from build123d import *

# Parameters (mm, degrees)
F0_R         = 1.75
F1_DEPTH     = 4
F2_W         = 50
F2_H         = 3
F3_DEPTH     = 35
F4_R         = 1.75
F5_DEPTH     = 3
F6_T1_DEPTH  = 4
F6_T6_DEPTH  = 28.6040226041
F6_T13_DEPTH = 28.6040226041
F6_S15_R     = 1.75
F6_T16_DEPTH = 16
F6_T19_DEPTH = 15.1872089077
F6_T26_DEPTH = 13.4620824192
F6_T30_DEPTH = 28.6040226041
F6_S32_R     = 1.75
F6_T33_DEPTH = 16
F7_R         = 3.25
F7_R_2       = 1.75
F8_DEPTH     = 2
F9_SIZE      = 2


# Not quite as in the source:
# - a fillet or chamfer that OpenCascade refuses, or shapes differently, is made with other operations: its cross-section is extruded or revolved along the edge and cut away or added


with BuildPart() as f1:
    # F0 (on Top) → F1 (new body)
    with BuildSketch(Plane.XY):
        Polygon((-4.0152793502, 1.5), (-25, 1.5), (-25, -1.5), (25, -1.5), (25, 1.5), (4.0152793502, 1.5), align=None)
        Polygon((-1.8013300137, 26.8055567119), (-4.0152793502, 1.5), (4.0152793502, 1.5), (6.1682275711, 26.10831077), align=None)
        with BuildLine():
            Line((-12.7594716927, 27.7642698822), (-1.8013300137, 26.8055567119))
            Line((-1.8013300137, 26.8055567119), (-1.4744959784, 30.5412868298))
            Line((-1.4744959784, 30.5412868298), (6.4950616064, 29.8440408878))
            Line((6.4950616064, 29.8440408878), (6.1682275711, 26.10831077))
            Line((6.1682275711, 26.10831077), (17.1263692501, 25.1495975997))
            ThreePointArc((17.1263692501, 25.1495975997), (14.9197400068, 31.6501177306), (21.2032032854, 28.8853277176))
            ThreePointArc((21.2032032854, 28.8853277176), (21.1996341163, 28.721755015), (21.1889334032, 28.5584936823))
            Line((21.1889334032, 28.5584936823), (23.8907614284, 59.4405293231))
            ThreePointArc((23.8907614284, 59.4405293231), (17.2823646489, 57.3569098221), (20.4818653459, 63.5030934763))
            Line((20.4818653459, 63.5030934763), (-9.4039755969, 66.1177657587))
            ThreePointArc((-9.4039755969, 66.1177657587), (-6.9660196192, 64.9154989194), (-5.9808096322, 62.3820356408))
            ThreePointArc((-5.9808096322, 62.3820356408), (-9.8943823348, 58.6356048099), (-13.46653975, 62.7088696761))
            Line((-13.46653975, 62.7088696761), (-16.1683677752, 31.8268340353))
            ThreePointArc((-16.1683677752, 31.8268340353), (-12.2690649548, 35.2464308309), (-8.6826376574, 31.5))
            ThreePointArc((-8.6826376574, 31.5), (-9.8991743788, 28.735209987), (-12.7594716927, 27.7642698822))
        make_face()
        Polygon((-8.9117487246, 34.4543766049), (-6.7764330273, 58.8611467081), (16.6341423778, 56.8129867535), (14.4988266805, 32.4062166503), align=None, mode=Mode.SUBTRACT)
        Polygon((-1.4744959784, 30.5412868298), (-1.8013300137, 26.8055567119), (6.1682275711, 26.10831077), (6.4950616064, 29.8440408878), align=None)
        with BuildLine():
            ThreePointArc((-16.1683677752, 31.8268340353), (-15.3053043191, 29.0895464637), (-12.7594716927, 27.7642698822))
            ThreePointArc((-12.7594716927, 27.7642698822), (-9.8991743788, 28.735209987), (-8.6826376574, 31.5))
            ThreePointArc((-8.6826376574, 31.5), (-12.2690649548, 35.2464308309), (-16.1683677752, 31.8268340353))
        make_face()
        with Locations((-12.4326376574, 31.5)):
            Circle(F0_R, mode=Mode.SUBTRACT)
        with BuildLine():
            ThreePointArc((21.2032032854, 28.8853277176), (14.9197400068, 31.6501177306), (17.1263692501, 25.1495975997))
            ThreePointArc((17.1263692501, 25.1495975997), (19.8636568217, 26.0126610559), (21.1889334032, 28.5584936823))
            ThreePointArc((21.1889334032, 28.5584936823), (21.1996341163, 28.721755015), (21.2032032854, 28.8853277176))
        make_face()
        with Locations((17.4532032854, 28.8853277176)):
            Circle(F0_R, mode=Mode.SUBTRACT)
        with BuildLine():
            ThreePointArc((-9.4039755969, 66.1177657587), (-12.1412631685, 65.2547023025), (-13.46653975, 62.7088696761))
            ThreePointArc((-13.46653975, 62.7088696761), (-9.8943823348, 58.6356048099), (-5.9808096322, 62.3820356408))
            ThreePointArc((-5.9808096322, 62.3820356408), (-6.9660196192, 64.9154989194), (-9.4039755969, 66.1177657587))
        make_face()
        with Locations((-9.7308096322, 62.3820356408)):
            Circle(F0_R, mode=Mode.SUBTRACT)
        with BuildLine():
            ThreePointArc((20.4818653459, 63.5030934763), (17.2823646489, 57.3569098221), (23.8907614284, 59.4405293231))
            ThreePointArc((23.8907614284, 59.4405293231), (23.9014621415, 59.6037906558), (23.9050313106, 59.7673633584))
            ThreePointArc((23.9050313106, 59.7673633584), (22.9198213236, 62.300826637), (20.4818653459, 63.5030934763))
        make_face()
        with Locations((20.1550313106, 59.7673633584)):
            Circle(F0_R, mode=Mode.SUBTRACT)
    extrude(amount=F1_DEPTH)

    # F2 (on face) → F3 (join)
    with BuildSketch(Plane.XY.offset(4)):
        Rectangle(F2_W, F2_H)
    extrude(amount=F3_DEPTH)

    # F4 (on face) → F5 (cut, through all)
    with BuildSketch(Plane.XZ.offset(1.5)):
        with Locations((-15, 34.5)):
            Circle(F4_R)
        with Locations((15, 34.5)):
            Circle(F4_R)
        with Locations((-15, 4.5)):
            Circle(F4_R)
        with Locations((15, 4.5)):
            Circle(F4_R)
        with Locations((0, 19.5)):
            Circle(F4_R)
    extrude(amount=-F5_DEPTH, mode=Mode.SUBTRACT)

    # F6: chamfer of 4 on 3 edges, made by hand

    # F6_s2 → F6_t1 (join)
    with BuildSketch(Plane.XY):
        Polygon((-7.6806040462, 1.5), (-3.6958252539, 5.151377029), (-4.0152793502, 1.5), align=None)
        Polygon((8.3805133545, 1.5), (4.3957345621, 5.848622971), (4.0152793502, 1.5), align=None)
    extrude(amount=F6_T1_DEPTH)


with BuildPart() as f6_tool4:
    # F6_s5 → F6_t6 (new body)
    with BuildSketch(Plane.YZ.offset(14.302011302)):
        Polygon((1.5, 8), (5.5, 4), (1.5, 4), align=None)
    extrude(amount=-F6_T6_DEPTH)

    split(bisect_by=Plane(origin=(-4.1150149256, 0.3600171562, 0), x_dir=(0, 0, 1), z_dir=(0.9961946981, -0.0871557427, 0)), keep=Keep.TOP)

    split(bisect_by=Plane(origin=(3.8545426591, -0.3372287857, 0), x_dir=(0, 0, 1), z_dir=(-0.9961946981, 0.0871557427, 0)), keep=Keep.TOP)


with BuildPart() as f1_1:
    add(f1.part)

    # F6_t3: union F6_tool4
    add(f6_tool4.part)


with BuildPart() as f6_tool11:
    # F6_s12 → F6_t13 (new body)
    with BuildSketch(Plane.YZ.offset(14.302011302)):
        Polygon((1.5, 8), (5.5, 4), (1.5, 4), align=None)
    extrude(amount=-F6_T13_DEPTH)

    split(bisect_by=Plane(origin=(3.8545426591, -0.3372287857, 0), x_dir=(0, 0, 1), z_dir=(0.9961946981, -0.0871557427, 0)), keep=Keep.TOP)

    # F6_s15 → F6_t16 (cut, symmetric)
    with BuildSketch(Plane.XZ.offset(-3.5)):
        with Locations((15, 4.5)):
            Circle(F6_S15_R)
    extrude(amount=F6_T16_DEPTH, both=True, mode=Mode.SUBTRACT)


with BuildPart() as f6_tool17:
    # F6_s18 → F6_t19 (new body)
    with BuildSketch(Plane.XY):
        Polygon((8.3805133545, 1.5), (4.3957345621, 5.848622971), (4.0152793502, 1.5), align=None)
    extrude(amount=F6_T19_DEPTH)

    split(bisect_by=Plane.XY.offset(4), keep=Keep.TOP)


with BuildPart() as f6_tool11_1:
    add(f6_tool11.part)

    # F6_t21: intersect F6_tool17
    add(f6_tool17.part, mode=Mode.INTERSECT)


with BuildPart() as f1_2:
    add(f1_1.part)

    # F6_t9: union F6_tool11
    add(f6_tool11_1.part)


with BuildPart() as f6_tool24:
    # F6_s25 → F6_t26 (new body)
    with BuildSketch(Plane.XY):
        Polygon((-7.6806040462, 1.5), (-3.6958252539, 5.151377029), (-4.0152793502, 1.5), align=None)
    extrude(amount=F6_T26_DEPTH)

    split(bisect_by=Plane.XY.offset(4), keep=Keep.TOP)


with BuildPart() as f6_tool28:
    # F6_s29 → F6_t30 (new body)
    with BuildSketch(Plane.YZ.offset(14.302011302)):
        Polygon((1.5, 8), (5.5, 4), (1.5, 4), align=None)
    extrude(amount=-F6_T30_DEPTH)

    split(bisect_by=Plane(origin=(-4.1150149256, 0.3600171562, 0), x_dir=(0, 0, 1), z_dir=(-0.9961946981, 0.0871557427, 0)), keep=Keep.TOP)

    # F6_s32 → F6_t33 (cut, symmetric)
    with BuildSketch(Plane.XZ.offset(-3.5)):
        with Locations((-15, 4.5)):
            Circle(F6_S32_R)
    extrude(amount=F6_T33_DEPTH, both=True, mode=Mode.SUBTRACT)


with BuildPart() as f6_tool24_1:
    add(f6_tool24.part)

    # F6_t34: intersect F6_tool28
    add(f6_tool28.part, mode=Mode.INTERSECT)


with BuildPart() as f1_3:
    add(f1_2.part)

    # F6_t22: union F6_tool24
    add(f6_tool24_1.part)

    # F7 (on face) → F8 (join)
    with BuildSketch(Plane.XY.offset(4)):
        with Locations((-9.7308096322, 62.3820356408)):
            Circle(F7_R)
        with Locations((-9.7308096322, 62.3820356408)):
            Circle(F7_R_2, mode=Mode.SUBTRACT)
        with Locations((20.1550313106, 59.7673633584)):
            Circle(F7_R)
        with Locations((20.1550313106, 59.7673633584)):
            Circle(F7_R_2, mode=Mode.SUBTRACT)
        with Locations((17.4532032854, 28.8853277176)):
            Circle(F7_R)
        with Locations((17.4532032854, 28.8853277176)):
            Circle(F7_R_2, mode=Mode.SUBTRACT)
        with Locations((-12.4326376574, 31.5)):
            Circle(F7_R)
        with Locations((-12.4326376574, 31.5)):
            Circle(F7_R_2, mode=Mode.SUBTRACT)
    extrude(amount=F8_DEPTH)

    # F9
    f9_edges = [f1_3.edges().sort_by_distance(p)[0] for p in [
        (6.168228, 26.108311, 2),
        (-1.80133, 26.805557, 2),
    ]]
    chamfer(f9_edges, length=F9_SIZE)


solid = f1_3.part
Check sheet for the modelled part. Datum: model origin and axes. Units: mm. A direction names the side the tool comes from. Round coordinates to 2 decimals unless told otherwise and drop trailing zeros. Loops run counter-clockwise (first coordinate to the right, second up) from the corner with the lowest first, then second, coordinate; pieces in that order, holes last.
1. Sectioned sample at B-B on z = 22. Record the boundary of the cut face in (x, y).
2. Scan lines: probe 1 along Z at (x, y) = (0, 0); probe 2 along Y at (x, z) = (-5.5, 8.5); probe 3 along Z at (x, y) = (0, 22). Record each from-to range of solid material in increasing order.
3. Sectioned sample at C-C on y = 11. Record the boundary of the cut face in (x, z), and give its area (3 significant figures).
4. Gauge pin test, flat ends, axial feed: pin 1 Ø5.5 at (x, z) = (15, 34.5) entering from +Y; pin 2 Ø7 at (x, y) = (-14, 30) entering from +Z; pin 3 Ø12 at (x, y) = (-5, 23) entering from +Z; pin 4 Ø3 at (x, y) = (-12.43, 31.5) entering from +Z (3 decimals). Record the tip position at first contact, or that the pin passes through.
5. Sectioned sample at A-A on x = 0. Record the boundary of the cut face in (y, z), and give its area (3 significant figures).
6. Set-up check for faces 1 (the flat face through (-11, 30, 6)), 2 (the flat face through (6.42, 3.64, 3.06)), 3 (the flat face through (15.58, 44.78, 1.97)), 4 (the cylindrical face through (17.76, 61.964, 4.986)): record each of +Z, -Z, +X, -X, +Y, -Y from which the full face is reachable in a straight line by a thin tool's end or side.
7. Mould release check, pull along Y, two halves, no side actions. Record for faces 5 (the flat face through (19, 27, 6)), 6 (the flat face through (-2.87, 25.88, 1.97)), 7 (the flat face through (0.5, 3, 6.5)): released by +Y, released by -Y, zero draft, split by the parting line, or undercut.
Recorded:
1. outline: (-25, -1.5) - (25, -1.5) - (25, 1.5) - (-25, 1.5) - close
2. probe 1: z = 0 to 17.75, 21.25 to 39
2. probe 2: y = -1.5 to 1.5
2. probe 3: z = 0 to 4
3. outline: (-3.18, 0) - (4.85, 0) - (4.85, 4) - (-3.18, 4) - close
3. area: 32.1 mm2
4. pin 1: stops at y = 1.5
4. pin 2: stops at z = 6
4. pin 3: stops at z = 4
4. pin 4: passes through
5. outline: (-1.5, 0) - (33.67, 0) - (33.67, 4) - (5.5, 4) - (1.5, 8) - (1.5, 17.75) - (-1.5, 17.75) - close; (-1.5, 21.25) - (1.5, 21.25) - (1.5, 39) - (-1.5, 39) - close; (58.27, 0) - (65.3, 0) - (65.3, 4) - (58.27, 4) - close
5. area: 271 mm2
6. face 1: +Z, +X, -X, +Y
6. face 2: +Z, -Z, +X
6. face 3: +Z, -Z
6. face 4: +Z
7. face 5: zero draft
7. face 6: undercut
7. face 7: released by +Y
